For this review, use the dimensioned drawing (mm, ordinates from the lowest corner) and the shaded views. Round coordinates to 2 decimals unless told otherwise and drop trailing zeros. Order: outer loops, then holes, each group sorted by start corner. A loop starts at its lowest first (then second) coordinate and runs counter-clockwise, first axis right, second up. Notation, with made-up numbers: (62, 24.5) -> (96, 24.5) arc R26 cw to (96, 59.5) -> close; hole circle Ø6 at (54.5, 84.25). An arc over 180 degrees is marked (long way). Answer in a Markdown table with one row per item.
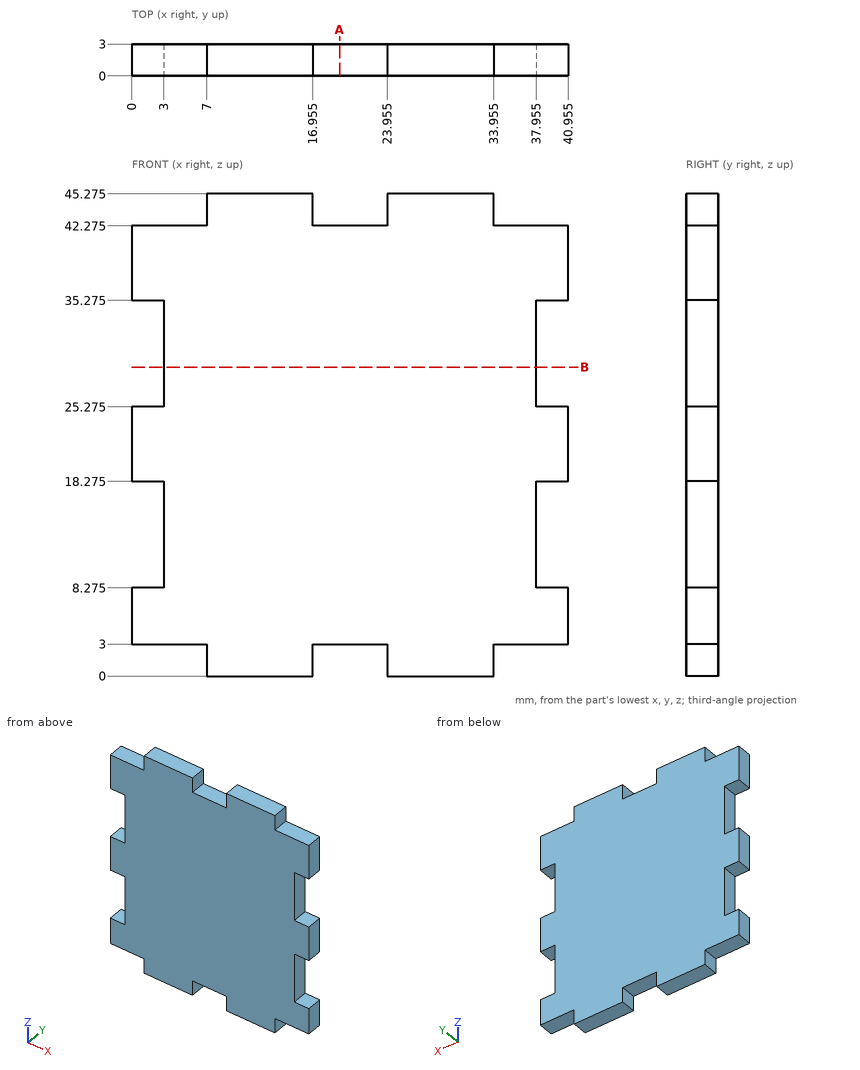
Q1. To check wall thickness, follow probe 1 along X at (y, z) = (1.65, 43.5) (1 decimal); probe 2 along Z at (x, y) = (18, 2.4) (1 decimal); probe 3 along X at (y, z) = (1.3, 32) (1 decimal). State the ranges of each line that lie inside material, in increasing order.
Answer key:
| item | result |
|---|---|
| probe 1 | x = 7 to 17, 24 to 34 |
| probe 2 | z = 3 to 42.3 |
| probe 3 | x = 3 to 38 |
Q2. Clearance check with flat-ended pins moving along their axes: pin 1 Ø0.9 at (x, y) = (21.5, 2) entering from -Z; pin 2 Ø1.5 at (y, z) = (2, 28) entering from -X; pin 3 Ø8 at (x, z) = (7.5, 33) entering from -Y; pin 4 Ø0.9 at (x, y) = (4, 1) entering from +Z (1 decimal). State where each tip first meets the part, or that it passes through.
Answer key:
| item | result |
|---|---|
| pin 1 | stops at z = 3 |
| pin 2 | stops at x = 3 |
| pin 3 | stops at y = 0 |
| pin 4 | stops at z = 42.3 |
Q3. Take a section at A-A, the plane x = 19.5. Write out the cut boundary in (y, z) (1 decimal), then the cut area to 3 significant figures.
Answer key:
| item | result |
|---|---|
| outline | (0, 3) -> (3, 3) -> (3, 42.3) -> (0, 42.3) -> close |
| area | 118 mm^2 |
Q4. Take a section at B-B, the plane z = 29. Write out the cut boundary in (x, y) (1 decimal).
Answer key:
| item | result |
|---|---|
| outline | (3, 0) -> (38, 0) -> (38, 3) -> (3, 3) -> close |
